Can you work these out from the drawing? Everything is in mm from the part's minimum corner. A direction names the side the tool comes from. Give positions to 0.01 mm unless a question says otherwise; leave off trailing zeros. Order: outer loops, then holes, each group sorted by start corner. A loop starts at its lowest first (then second) coordinate and runs counter-clockwise, first axis right, second up. Notation, with made-up numbers: (58, 49) - (83, 49) arc R20 ccw to (83, 73) - close; hole circle Ø10 at (25, 46). An arc over 180 degrees is marked (long way). Answer as a JSON object with one key per item and string values.
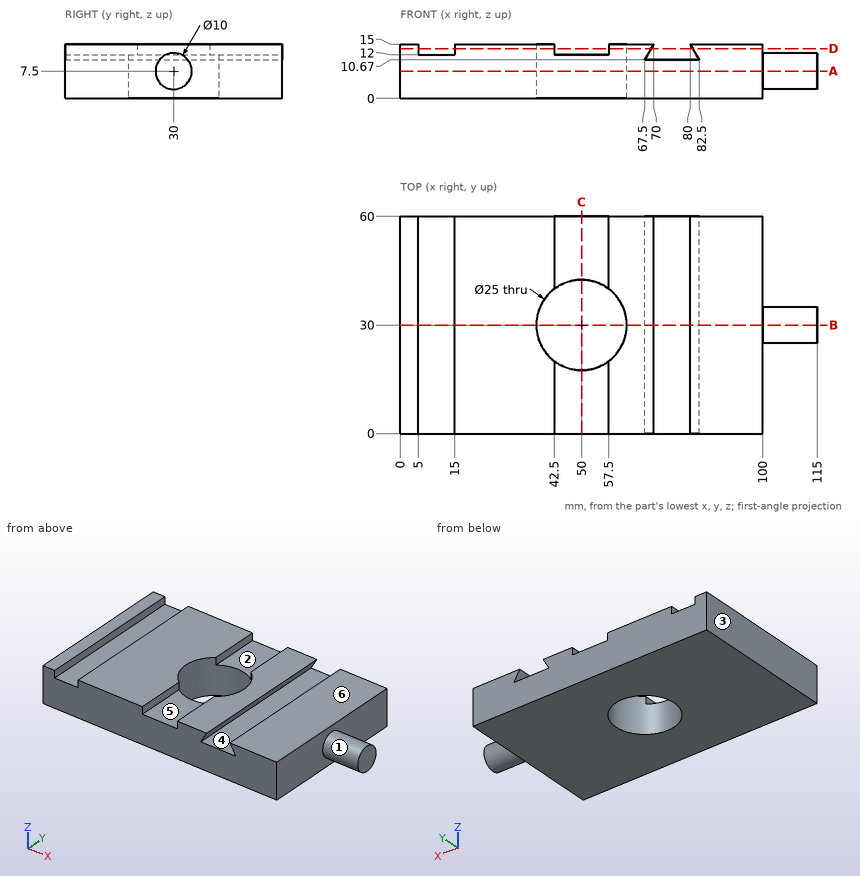
Q1. We'd pull the mould along X, two halves only. Please class the marked faces 1, 2 and 3: released by +X, released by -X, zero draft, split by the parting line, or undercut.
Recorded:
{"face 1": "zero draft", "face 2": "undercut", "face 3": "released by -X"}
Q2. If we section it at C-C, the plane x = 50: Please give me the cut outline in (y, z).
Recorded:
{"outline": "(0, 0) - (17.5, 0) - (17.5, 12) - (0, 12) - close; (42.5, 0) - (60, 0) - (60, 12) - (42.5, 12) - close"}
Q3. If we section it at A-A, the plane z = 7.5: Please give me the cut outline in (x, y), then the cut area to 3 significant figures.
Recorded:
{"outline": "(0, 0) - (100, 0) - (100, 25) - (115, 25) - (115, 35) - (100, 35) - (100, 60) - (0, 60) - close; hole circle Ø25 at (50, 30)", "area": "5,660 mm^2"}
Q4. If we section it at B-B, the plane y = 30: Please give me the cut outline in (x, z), then the cut area to 3 significant figures.
Recorded:
{"outline": "(0, 0) - (37.5, 0) - (37.5, 15) - (15, 15) - (15, 12) - (5, 12) - (5, 15) - (0, 15) - close; (62.5, 0) - (100, 0) - (100, 2.5) - (115, 2.5) - (115, 12.5) - (100, 12.5) - (100, 15) - (80, 15) - (82.5, 10.67) - (67.5, 10.67) - (70, 15) - (62.5, 15) - close", "area": "1,190 mm^2"}
Q5. I'm going to push flat-ended pins straight in: pin 1 Ø1.5 at (y, z) = (40, 14) entering from -X; pin 2 Ø3.5 at (y, z) = (38.5, 14) entering from +X; pin 3 Ø4.5 at (x, y) = (52.5, 11) entering from +Z; pin 4 Ø1.5 at (x, z) = (12.5, 13.5) entering from -Y. Where does each tip first touch, or does it pass through?
Recorded:
{"pin 1": "stops at x = 0", "pin 2": "stops at x = 100", "pin 3": "stops at z = 12", "pin 4": "passes through"}
Q6. I need wall thicknesses on L1, parallel to Y at x = 50, z = 5.5; L2, parallel to X at y = 20, z = 9.75; L3, parallel to X at y = 30, z = 3.5. Which ranges of each line are inside material? Lowest first, please.
Recorded:
{"L1": "y = 0 to 17.5, 42.5 to 60", "L2": "x = 0 to 42.5, 57.5 to 100", "L3": "x = 0 to 37.5, 62.5 to 115"}
Q7. Which directions (+Z, -Z, +X, -X, +Y, -Y) give clear straight access to the entire face, cutting with the end or side of a thin tool? Please do the marked faces 4, 5 and 6.
Recorded:
{"face 4": "+Y, -Y", "face 5": "+Z, +Y, -Y", "face 6": "+Z, +X, -X, +Y, -Y"}
Q8. If we section it at D-D, the plane z = 13.75: Please give me the cut outline in (x, y).
Recorded:
{"outline": "(0, 0) - (5, 0) - (5, 60) - (0, 60) - close; (15, 0) - (42.5, 0) - (42.5, 20) arc R12.5 cw to (42.5, 40) - (42.5, 60) - (15, 60) - close; (57.5, 0) - (69.28, 0) - (69.28, 60) - (57.5, 60) - (57.5, 40) arc R12.5 cw to (57.5, 20) - close; (80.72, 0) - (100, 0) - (100, 60) - (80.72, 60) - close"}
